Read the model definition and answer for the solid it produces. Units are mm, in the model's axes. Face numbers are marked on the shaded views. A direction names the side the tool comes from. Coordinates: 2 decimals unless noted, no trailing zeros. Loops run counter-clockwise (first coordinate to the right, second up) from the corner with the lowest first, then second, coordinate; pieces in that order, holes last.
Q1. Section C-C (z = 7.5) is taken. Give the vertices of the cut face in (x, y), then the cut area to 3 significant figures.
Q2. Section D-D (y = 32) is taken. Give the vertices of the cut face in (x, z), then the cut area to 3 significant figures.
Q3. Section B-B (z = 24) is taken. Give the vertices of the cut face in (x, y).
Q4. Straight lines are drawn through the part: line 1 (Z direction, x = 6.5, y = 20); line 2 (Z direction, x = 38.5, y = 45). For each, find the intervals that lie inside material, in ascending order.
Q5. Flat-ended cylindrical pins translate along their axes: P1, Ø1.5, axis at x = 16.5, y = 18, coming from the +Z side; P2, Ø5, axis at y = 35, z = 57.5, coming from the +X side. Find the tip coordinate at first contact, or state that the pin passes through.
Q6. Section A-A (x = 27) is taken. Give the vertices of the cut face in (y, z), then the cut area to 3 significant figures.
Q7. The mould has two halves that part along Z. Classify the marked faces 1, 2, 3 and 4: pulls with the +Z half, pulls with the -Z half, needs draft (parallel to the pull), parting line crosses it, or undercut.
Q8. Which of the six approach directions +Z, -Z, +X, -X, +Y, -Y give full straight-line access (tool end or side, diameter ignored) to the marked faces 5 and 6?
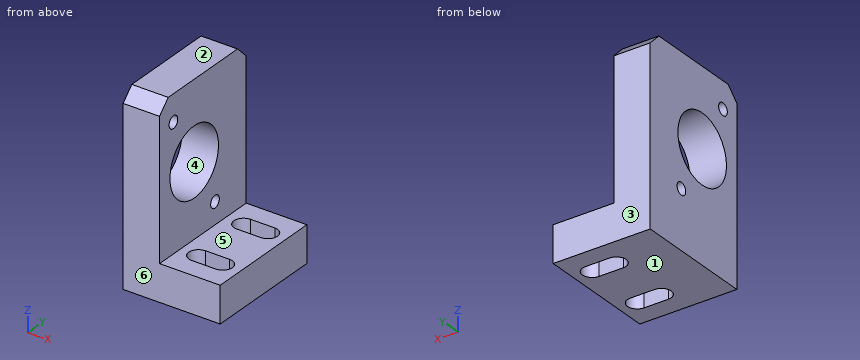
from build123d import *

# Parameters (mm, degrees)
F0_W      = 40
F0_H      = 50
F1_DEPTH  = 15
F2_W      = 15
F2_H      = 50
F3_DEPTH  = 62
F4_R      = 14
F5_DEPTH  = 15
F6_SIZE   = 5
F7_R      = 2.5
F8_DEPTH  = 15
F10_DEPTH = 15


with BuildPart() as f1:
    # F0 (on Top) → F1 (new body)
    with BuildSketch(Plane.XY):
        with Locations((20, 25)):
            Rectangle(F0_W, F0_H)
    extrude(amount=F1_DEPTH)

    # F2 (on face) → F3 (join)
    with BuildSketch(Plane.XY.offset(15)):
        with Locations((7.5, 25)):
            Rectangle(F2_W, F2_H)
    extrude(amount=F3_DEPTH)

    # F4 (on face) → F5 (cut, through all)
    with BuildSketch(Plane.YZ.offset(15)):
        with Locations((20, 45)):
            Circle(F4_R)
    extrude(amount=-F5_DEPTH, mode=Mode.SUBTRACT)

    # F6
    f6_edges = [f1.edges().sort_by_distance(p)[0] for p in [
        (7.5, 50, 77),
        (7.5, 0, 77),
    ]]
    chamfer(f6_edges, length=F6_SIZE)

    # F7 (on face) → F8 (cut, through all)
    with BuildSketch(Plane.YZ.offset(15)):
        with Locations((8, 66)):
            Circle(F7_R)
        with Locations((32, 24)):
            Circle(F7_R)
    extrude(amount=-F8_DEPTH, mode=Mode.SUBTRACT)

    # F9 (on face) → F10 (cut, through all)
    with BuildSketch(Plane.XY.offset(15)):
        with BuildLine():
            Line((32.5, 42), (22.5, 42))
            ThreePointArc((22.5, 42), (18.5, 38), (22.5, 34))
            Line((22.5, 34), (32.5, 34))
            ThreePointArc((32.5, 34), (36.5, 38), (32.5, 42))
        make_face()
        with BuildLine():
            Line((32.5, 16), (22.5, 16))
            ThreePointArc((22.5, 16), (18.5, 12), (22.5, 8))
            Line((22.5, 8), (32.5, 8))
            ThreePointArc((32.5, 8), (36.5, 12), (32.5, 16))
        make_face()
    extrude(amount=-F10_DEPTH, mode=Mode.SUBTRACT)


solid = f1.part
Numbers:
1. outline: (0, 0) - (40, 0) - (40, 50) - (0, 50) - close; hole (22.5, 8) - (32.5, 8) arc R4 ccw to (32.5, 16) - (22.5, 16) arc R4 ccw to start; hole (22.5, 34) - (32.5, 34) arc R4 ccw to (32.5, 42) - (22.5, 42) arc R4 ccw to start
1. area: 1,740 mm2
2. outline: (0, 0) - (40, 0) - (40, 15) - (15, 15) - (15, 21.5) - (0, 21.5) - close; (0, 26.5) - (15, 26.5) - (15, 37.79) - (0, 37.79) - close; (0, 52.21) - (15, 52.21) - (15, 77) - (0, 77) - close
2. area: 1,240 mm2
3. outline: (0, 0) - (15, 0) - (15, 29.5) - (0, 29.5) - close; (0, 34.5) - (15, 34.5) - (15, 50) - (0, 50) - close
4. line 1: z = 0 to 31, 59 to 77
4. line 2: z = 0 to 15
5. P1: stops at z = 15
5. P2: stops at x = 15
6. outline: (0, 0) - (8, 0) - (8, 15) - (0, 15) - close; (16, 0) - (34, 0) - (34, 15) - (16, 15) - close; (42, 0) - (50, 0) - (50, 15) - (42, 15) - close
6. area: 510 mm2
7. face 1: pulls with the -Z half
7. face 2: pulls with the +Z half
7. face 3: needs draft
7. face 4: undercut
8. face 5: +Z, +X, +Y, -Y
8. face 6: +Z, -Z, +X, -X, -Y
